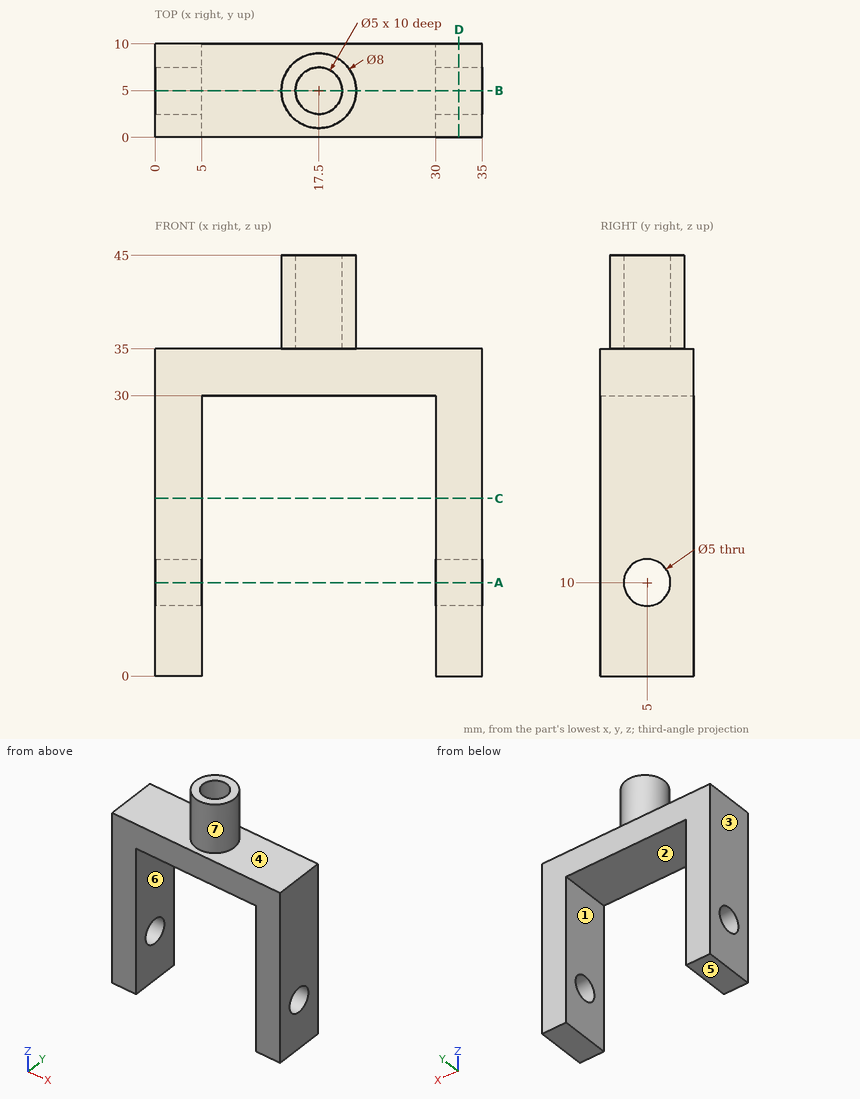
Here's the drawing with two shaded views (mm, measured from the low corner). I have some questions. A direction names the side the tool comes from. Coordinates: 2 decimals unless noted, no trailing zeros. Order: outer loops, then holes, each group sorted by start corner. A loop starts at its lowest first (then second) coordinate and runs counter-clockwise, first axis right, second up.
Item 1: If we section it at C-C, the plane z = 19: List the corners of the cut face in (x, y) for me, then the cut area to 3 significant figures.
Response values:
outline: (0, 0) - (5, 0) - (5, 10) - (0, 10) - close; (30, 0) - (35, 0) - (35, 10) - (30, 10) - close
area: 100 mm2
Item 2: I'm going to push flat-ended pins straight in: pin 1 Ø2.5 at (x, y) = (18, 5.5) entering from +Z; pin 2 Ø5 at (x, y) = (17.5, 2.5) entering from -Z; pin 3 Ø3 at (y, z) = (4, 40.5) entering from -X. Where does each tip first touch, or does it pass through?
Response values:
pin 1: stops at z = 35
pin 2: stops at z = 30
pin 3: stops at x = 13.5
Item 3: If we section it at B-B, the plane y = 5: List the corners of the cut face in (x, z) for me, then the cut area to 3 significant figures.
Response values:
outline: (0, 0) - (5, 0) - (5, 7.5) - (0, 7.5) - close; (0, 12.5) - (5, 12.5) - (5, 30) - (30, 30) - (30, 12.5) - (35, 12.5) - (35, 35) - (21.5, 35) - (21.5, 45) - (20, 45) - (20, 35) - (15, 35) - (15, 45) - (13.5, 45) - (13.5, 35) - (0, 35) - close; (30, 0) - (35, 0) - (35, 7.5) - (30, 7.5) - close
area: 455 mm2
Item 4: If we section it at A-A, the plane z = 10: List the corners of the cut face in (x, y) for me.
Response values:
outline: (0, 0) - (5, 0) - (5, 2.5) - (0, 2.5) - close; (0, 7.5) - (5, 7.5) - (5, 10) - (0, 10) - close; (30, 0) - (35, 0) - (35, 2.5) - (30, 2.5) - close; (30, 7.5) - (35, 7.5) - (35, 10) - (30, 10) - close
Item 5: If we section it at D-D, the plane x = 32.5: List the corners of the cut face in (y, z) for me, then the cut area to 3 significant figures.
Response values:
outline: (0, 0) - (10, 0) - (10, 35) - (0, 35) - close; hole circle Ø5 at (5, 10)
area: 330 mm2
Item 6: I need wall thicknesses on probe 1 along X at (y, z) = (7.5, 9); probe 2 along X at (y, z) = (5, 43); probe 3 along Y at (x, z) = (3.35, 10). Which ranges of each line are inside material? Lowest first, please.
Response values:
probe 1: x = 0 to 5, 30 to 35
probe 2: x = 13.5 to 15, 20 to 21.5
probe 3: y = 0 to 2.5, 7.5 to 10
Item 7: Thinking about a two-plate mould opening in X: for the marked faces 1, 2, 3 and 4, which applies, pulls with the +X half, pulls with the -X half, needs draft (parallel to the pull), parting line crosses it, or undercut?
Response values:
face 1: undercut
face 2: undercut
face 3: pulls with the -X half
face 4: needs draft
Item 8: Which directions (+Z, -Z, +X, -X, +Y, -Y) give clear straight access to the entire face, cutting with the end or side of a thin tool? Please do the marked faces 5, 6 and 7.
Response values:
face 5: -Z, +X, -X, +Y, -Y
face 6: -Z, +Y, -Y
face 7: +Z
